Autodesk Inventor part; units mm, degrees
ref_plane "Work Plane1" through (0, 10, 0) normal (0, -1, 0) x (1, 0, 0)
ref_plane "YZ Plane" through (0, 0, 0) normal (1, 0, 0) x (0, 1, 0)
ref_plane "XZ Plane" through (0, 0, 0) normal (0, 1, 0) x (-1, 0, 0)
sketch "Sketch1" plane through (0, 0, 0) normal (0, 1, 0) x (-1, 0, 0)
  circle A0 centre (0, 0) radius 21
  line L0 (10, 10) -> (-10, 10)
  line L1 (-10, 10) -> (-10, -10)
  line L2 (-10, -10) -> (10, -10)
  line L3 (10, -10) -> (10, 10)
  line L4 (10, 10) -> (-10, -10) construction
  line L5 (-10, 10) -> (10, -10) construction
  dimension "d0" = 42
  dimension "d1" = 20
  dimension "d2" = 20
extrude "Extrusion1" add sketch "Sketch1" along normal blind 90 contours A0 | L3 L2 L1 L0
extrude "Extrusion2" add sketch "Sketch1" against normal blind 20 contours L3 L2 L1 L0
ref_plane "Work Plane1" through (0, 10, 0) normal (0, -1, 0) x (1, 0, 0)
sketch "Sketch2" plane through (0, 10, 0) normal (0, -1, 0) x (1, 0, 0)
  circle A0 centre (-25, 15) radius 1.5
  circle A1 centre (-25, -15) radius 1.5
  circle A2 centre (0, 0) radius 21
  line L0 (-15.6197, 14.0366) -> (-22.942, 18.43)
  arc A3 (-22.942, 18.43) -> (-27.058, 11.57) centre (-25, 15) ccw
  line L1 (-27.058, 11.57) -> (-19.7357, 7.1766)
  line L2 (-19.7357, -7.1766) -> (-27.058, -11.57)
  arc A4 (-27.058, -11.57) -> (-22.942, -18.43) centre (-25, -15) ccw
  line L3 (-22.942, -18.43) -> (-15.6197, -14.0366)
  line L4 (-25, 15) -> (0, 0) construction
  line L5 (0, 0) -> (-25, -15) construction
  point P0 (-21, 0)
  dimension "d8" = 3
  dimension "d9" = 30
  dimension "d10" = 15
  dimension "d11" = 4
  dimension "d12" = 4
  dimension "d13" = 4
extrude "Extrusion3" add sketch "Sketch2" along normal blind 3 contours A2 L1 A3 L0 | L3 A4 L2 A2
pattern_linear "Rectangular Pattern2" count 2 spacing 8 along (0, 1, 0) of "Extrusion3"
pattern_linear "Rectangular Pattern1" count 2 spacing 50 along (0, 1, 0) of "Extrusion3", "Rectangular Pattern2"
properties part number "MockPitchMotor" material "ABS Plastic"
Geometry: final body of the model. Coordinates: model frame, mm. A direction names the side the tool comes from. Round coordinates to 2 decimals unless told otherwise and drop trailing zeros. Loops run counter-clockwise (first coordinate to the right, second up) from the corner with the lowest first, then second, coordinate; pieces in that order, holes last.
Q1. Access query for faces 4 (the flat face through (-23.448, 16.521, 9.404)), 5 (the flat face through (-19.332, 16.521, -16.264)), 6 (the flat face through (-19.23, 16.521, 16.203)). Directions: +Z, -Z, +X, -X, +Y, -Y. A direction counts if a zero-diameter tool reaches every point of the face in a straight line with its end or side. Return the directions, or none.
Q2. Pull-direction query (Y, two-part tool) for faces 1 (the flat face through (-22, 7, 13)), 2 (the cylindrical face through (-28.474, 16.521, 16.982)), 3 (the flat face through (-22, 10, 13)); classes: released by +Y, released by -Y, zero draft, split by the parting line, or undercut.
Q3. Section A-A on x = 0. Return loops of the section in (y, z), plus the area to 3 significant figures.
Q4. Section B-B on z = 0. Return loops of the section in (x, y).
Q5. Section C-C on y = -11.5. Return loops of the section in (x, z), plus the area to 3 significant figures.
Q6. Material intervals for L1, parallel to Y at x = -26, z = -18; L2, parallel to Z at x = -25, y = 67; L3, parallel to Y at x = -6, z = -13, sorted ascending.
Q7. Pin query (flat end, axial travel): P1, Ø2.5, axis at x = -25, z = -15, coming from the -Y side; P2, Ø13, axis at x = -22, z = 14, coming from the +Y side; P3, Ø6, axis at x = -21, z = 15, coming from the +Y side; P4, Ø5, axis at y = 3, z = 6, coming from the -X side. Return the tip coordinate at first contact, or that it passes through.
Q8. Section D-D on x = -25. State how many separate pieces and enclosed holes the cut face has, plus the area to 3 significant figures.
Evaluation:
1. face 4: -X, +Y, -Y
1. face 5: -Z, +Y, -Y
1. face 6: +Z, +Y, -Y
2. face 1: released by -Y
2. face 2: zero draft
2. face 3: undercut
3. outline: (-20, -10) - (0, -10) - (0, -21) - (90, -21) - (90, 21) - (0, 21) - (0, 10) - (-20, 10) - close
3. area: 4,180 mm2
4. outline: (-21, 0) - (-10, 0) - (-10, -20) - (10, -20) - (10, 0) - (21, 0) - (21, 90) - (-21, 90) - close
5. outline: (-10, -10) - (10, -10) - (10, 10) - (-10, 10) - close
5. area: 400 mm2
6. L1: y = 7 to 10, 15 to 18, 57 to 60, 65 to 68
6. L2: z = -19 to -16.5, -13.5 to -10.34, 10.34 to 13.5, 16.5 to 19
6. L3: y = 0 to 90
7. P1: passes through
7. P2: stops at y = 90
7. P3: stops at y = 68
7. P4: stops at x = -20.71
8. separate pieces: 16
8. enclosed holes: 0
8. area: 136 mm2
